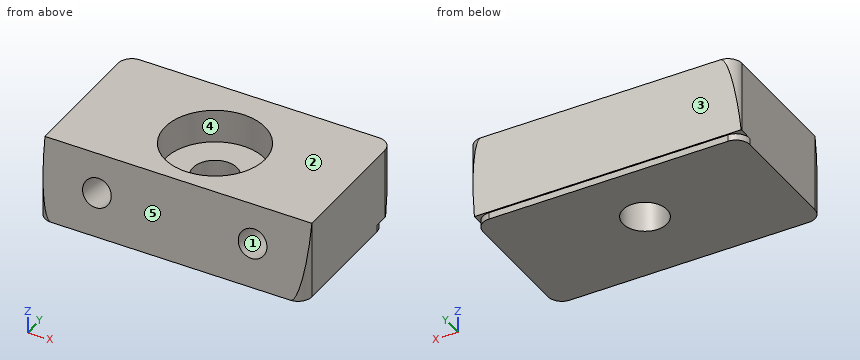
from build123d import *

# Parameters (mm, degrees)
F0_W           = 60.96
F0_H           = 35.56
F1_DEPTH       = 17.78
F2_R           = 3.175
F4_DEPTH       = 60.961
F6_D           = 10.0838
F6_DEPTH       = 23.2918
F6_CBORE_D     = 22.86
F6_CBORE_DEPTH = 7.62
F6_TIP         = 3.0294791551
F7_T1_DEPTH    = 9.4615000248
F9_D           = 6.5278
F9_DEPTH       = 23.2833333333
F9_TIP         = 1.9611489744


# Not quite as in the source:
# - a fillet or chamfer that OpenCascade refuses, or shapes differently, is made with other operations: its cross-section is extruded or revolved along the edge and cut away or added
# - a feature names something its author has since deleted; it is built from what else it names


with BuildPart() as f1:
    # F0 (on Top) → F1 (new body)
    with BuildSketch(Plane.XY):
        with Locations((30.48, 17.78)):
            Rectangle(F0_W, F0_H)
    extrude(amount=F1_DEPTH)

    # F2
    f2_edges = [f1.edges().sort_by_distance(p)[0] for p in [
        (0, 0, 8.89),
        (60.96, 0, 8.89),
        (60.96, 35.56, 8.89),
        (0, 35.56, 8.89),
    ]]
    fillet(f2_edges, radius=F2_R)

    # F3 (on face) → F4 (cut, through all)
    with BuildSketch(Plane.YZ.offset(60.96)):
        Polygon((0, 17.78), (0, 0), (3.135093717, 17.78), align=None)
        Polygon((32.424906283, 1.524), (32.424906283, 0), (35.56, 0), (35.56, 17.78), (32.6936286016, 1.524), align=None)
    extrude(amount=-F4_DEPTH, mode=Mode.SUBTRACT)

    # F6
    with Locations(Plane.XY.offset(17.78)):
        with Locations((30.4801253996, 17.78)):
            CounterBoreHole(F6_D / 2, F6_CBORE_D / 2, F6_CBORE_DEPTH, depth=F6_DEPTH)
            with Locations((0, 0, -(F6_DEPTH + F6_TIP / 2))):  # 118° drill point
                Cone(0, F6_D / 2, F6_TIP, mode=Mode.SUBTRACT)

    # F7: fillet of radius 3.175 on 2 edges, made by hand

    # F7_s2 → F7_t1 (cut)
    with BuildSketch(Plane.XY.offset(-7.9375000248)):
        with BuildLine():
            ThreePointArc((57.785, 32.424906283), (60.0300640303, 31.4949703133), (60.96, 29.249906283))
            Line((60.96, 29.249906283), (61.2775, 29.249906283))
            ThreePointArc((61.2775, 29.249906283), (61.2775, 32.385), (61.277224121, 32.4288969113))
            Line((61.277224121, 32.4288969113), (60.9597492009, 32.742406283))
            Line((60.9597492009, 32.742406283), (57.785, 32.742406283))
            Line((57.785, 32.742406283), (57.785, 32.424906283))
        make_face()
        with BuildLine():
            ThreePointArc((0, 29.249906283), (0.9299359697, 31.4949703133), (3.175, 32.424906283))
            Line((3.175, 32.424906283), (3.175, 32.742406283))
            Line((3.175, 32.742406283), (0.0002507991, 32.742406283))
            Line((0.0002507991, 32.742406283), (-0.317224121, 32.4288969113))
            ThreePointArc((-0.317224121, 32.4288969113), (-0.3175, 32.385), (-0.3175, 29.249906283))
            Line((-0.3175, 29.249906283), (0, 29.249906283))
        make_face()
    extrude(amount=F7_T1_DEPTH, mode=Mode.SUBTRACT)

    # F9
    with Locations(Plane(origin=(0, 0, 0), x_dir=(1, 0, 0), z_dir=(0, -0.984807753, 0.1736481777))):
        with Locations((12.7, 9.525), (48.26, 9.525)):
            Hole(F9_D / 2, depth=F9_DEPTH)
            with Locations((0, 0, -(F9_DEPTH + F9_TIP / 2))):  # 118° drill point
                Cone(0, F9_D / 2, F9_TIP, mode=Mode.SUBTRACT)


solid = f1.part
For this review, take the finished solid that the model builds, in its own axes (mm). Face numbers are marked on the shaded views. A direction names the side the tool comes from. Give positions to 0.01 mm unless a question says otherwise; leave off trailing zeros. Loops run counter-clockwise (first coordinate to the right, second up) from the corner with the lowest first, then second, coordinate; pieces in that order, holes last.
Item 1: Take a section at B-B, the plane y = 14. Give the number of separate pieces and of enclosed holes in the cut face, and give its area (3 significant figures).
Item 2: Insertion check: pin 1 (7 mm diameter, centred on x = 29, y = 15, fed in from +Z); pin 2 (0.5 mm diameter, centred on x = 23.5, z = 0.5, fed in from +Y); pin 3 (2 mm diameter, centred on x = 31, z = 11.5, fed in from -Y). Each pin has a flat end and moves straight along its axis. Give the tip position at first contact, or say it passes through.
Item 3: Draft analysis for pull direction Y (two halves, no side actions). For the marked faces 1, 2 and 3, state which applies: +Y half, -Y half, draft (parallel to the pull), parting line (faces both ways), or undercut.
Item 4: Tool access review of the marked faces 4 and 5: name each direction out of +Z, -Z, +X, -X, +Y, -Y from which nothing blocks a thin tool from reaching the whole face with its end or side.
Item 5: Take a section at A-A, the plane x = 52.5. State the section outline as (y, z) points, and give its area (3 significant figures).
Item 6: Take a section at C-C, the plane x = 31.5. State the section outline as (y, z) points.
Item 7: Take a section at D-D, the plane z = 14. State the section outline as (x, y) points (3 decimals).
Item 8: For line 1 along X through (y, z) = (17.5, 7); line 2 along Z through (x, y) = (39, 16.5); line 3 along X through (y, z) = (23, 10.5), list the stretches that pass through material, from the lowest coordinate up.
Calculated:
1. separate pieces: 2
1. enclosed holes: 2
1. area: 784 mm2
2. pin 1: stops at z = 10.16
2. pin 2: stops at y = 32.42
2. pin 3: stops at y = 1.85
3. face 1: undercut
3. face 2: draft
3. face 3: +Y half
4. face 4: +Z
4. face 5: +Z, +X, -X, -Y
5. outline: (0, 0) - (32.42, 0) - (32.42, 1.52) - (32.69, 1.52) - (35.56, 17.78) - (3.14, 17.78) - close
5. area: 576 mm2
6. outline: (0, 0) - (12.84, 0) - (12.84, 10.16) - (6.4, 10.16) - (6.4, 17.78) - (3.14, 17.78) - close; (22.72, 0) - (32.42, 0) - (32.42, 1.52) - (32.69, 1.52) - (35.56, 17.78) - (29.16, 17.78) - (29.16, 10.16) - (22.72, 10.16) - close
7. outline: (0, 3.175) arc R3.175 ccw to (0.08, 2.469) - (60.88, 2.469) arc R3.175 ccw to (60.96, 3.175) - (60.96, 32.385) arc R3.175 ccw to (59.731, 34.893) - (1.229, 34.893) arc R3.175 ccw to (0, 32.385) - close; hole circle Ø22.86 at (30.48, 17.78)
8. line 1: x = 0 to 9.46, 15.94 to 25.45, 35.51 to 45.02, 51.5 to 60.96
8. line 2: z = 0 to 10.16
8. line 3: x = 0 to 20.31, 40.65 to 60.96
